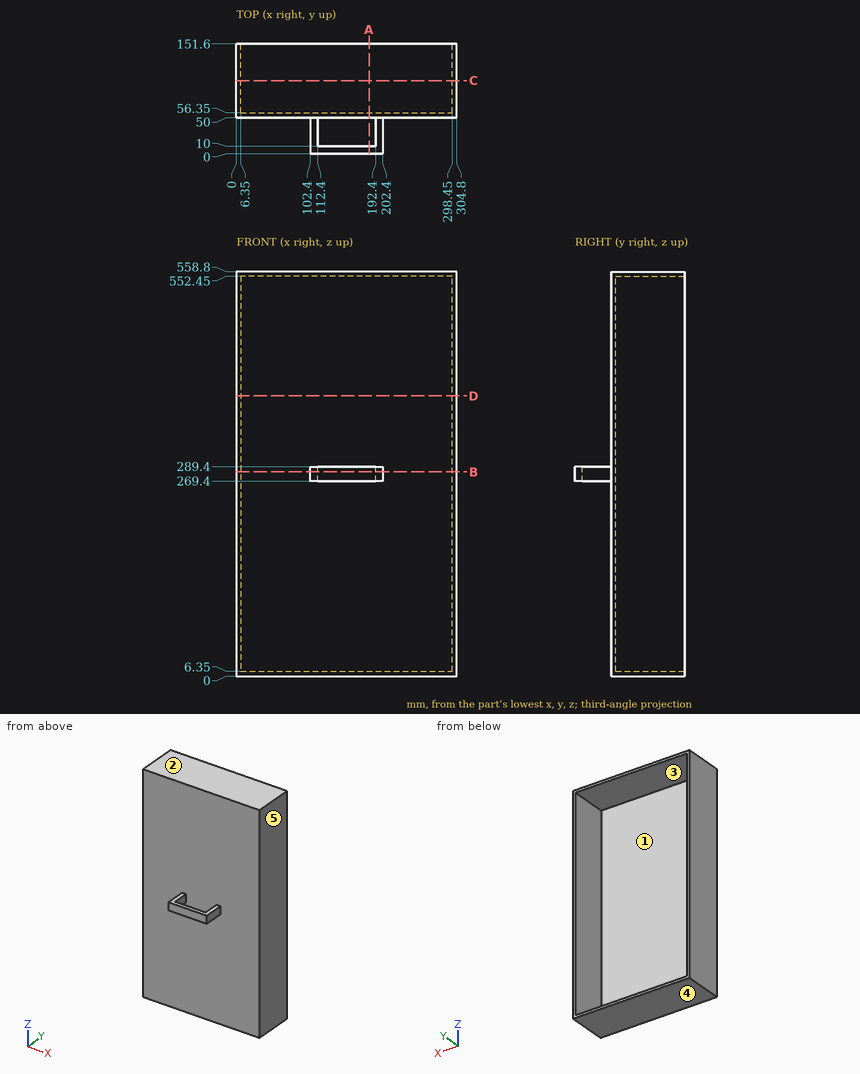
Study the drawing (mm; zero at the part's minimum x, y, z) and answer. A direction names the side the tool comes from. Round coordinates to 2 decimals unless told otherwise and drop trailing zeros. Write each loop counter-clockwise with the first axis right and the second up, starting at its lowest first coordinate (ties: lowest second). Pieces come first, ordered by that corner, then holes.
Q1. Find section A-A on x = 183.5. Determine the outline of the cut face in (y, z), and give its area (3 significant figures).
Values:
outline: (0, 269.4) - (10, 269.4) - (10, 289.4) - (0, 289.4) - close; (50, 0) - (151.6, 0) - (151.6, 6.35) - (56.35, 6.35) - (56.35, 552.45) - (151.6, 552.45) - (151.6, 558.8) - (50, 558.8) - close
area: 4,960 mm2
Q2. Find section D-D on z = 387. Determine the outline of the cut face in (x, y).
Values:
outline: (0, 50) - (304.8, 50) - (304.8, 151.6) - (298.45, 151.6) - (298.45, 56.35) - (6.35, 56.35) - (6.35, 151.6) - (0, 151.6) - close
Q3. Find section C-C on y = 101. Determine the outline of the cut face in (x, z), and give its area (3 significant figures).
Values:
outline: (0, 0) - (304.8, 0) - (304.8, 558.8) - (0, 558.8) - close; hole (6.35, 6.35) - (298.45, 6.35) - (298.45, 552.45) - (6.35, 552.45) - close
area: 10,800 mm2
Q4. Flat-ended cylindrical pins translate along their axes: P1, Ø22, axis at y = 22.5, z = 281.5, coming from the -X side; P2, Ø4, axis at x = 228, z = 316.5, coming from the -Y side; P3, Ø12, axis at y = 108.5, z = 174, coming from the -X side; P4, Ø6, axis at y = 29.5, z = 279, coming from the +X side. Find the tip coordinate at first contact, or state that the pin passes through.
Values:
P1: stops at x = 102.4
P2: stops at y = 50
P3: stops at x = 0
P4: stops at x = 202.4
Q5. Find section B-B on z = 282. Determine the outline of the cut face in (x, y).
Values:
outline: (0, 50) - (102.4, 50) - (102.4, 0) - (202.4, 0) - (202.4, 50) - (304.8, 50) - (304.8, 151.6) - (298.45, 151.6) - (298.45, 56.35) - (6.35, 56.35) - (6.35, 151.6) - (0, 151.6) - close; hole (112.4, 10) - (192.4, 10) - (192.4, 50) - (112.4, 50) - close
Q6. Straight lines are drawn through the part: line 1 (Z direction, x = 154.5, y = 101.5); line 2 (X direction, y = 89, z = 483); line 3 (Y direction, x = 127.5, z = 142.5). For each, find the intervals that lie inside material, in ascending order.
Values:
line 1: z = 0 to 6.35, 552.45 to 558.8
line 2: x = 0 to 6.35, 298.45 to 304.8
line 3: y = 50 to 56.35
Q7. A tool of negligible diameter and unlimited length cuts with its end or side. For the marked faces 1 and 2, from which of +Z, -Z, +X, -X, +Y, -Y can it reach the whole face along a straight path? Write none if from no direction.
Values:
face 1: +Y
face 2: +Z, +X, -X, +Y, -Y
Q8. The mould has two halves that part along X. Classify the marked faces 3, 4 and 5: released by +X, released by -X, zero draft, split by the parting line, or undercut.
Values:
face 3: undercut
face 4: zero draft
face 5: released by +X
